Model file for the job. Use its own axes, mm. Give positions to 0.01 mm unless a question says otherwise; leave off trailing zeros. Write each loop counter-clockwise with the first axis right and the second up, starting at its lowest first coordinate (ties: lowest second). Pieces come first, ordered by that corner, then holes. Notation, with made-up numbers: (36.5, 9.25) - (81.5, 9.25) arc R21 cw to (81.5, 44.25) - close; hole circle Ø8 at (54.5, 66). An arc over 180 degrees is marked (long way). Use CSV: the item, a comma, the result in double quotes.
Solid Edge part; units mm, degrees
sketch "Sketch1" plane through (0, 0, 0) normal (0, 0, 1) x (1, 0, 0)
  line L0 (13.5, 20.7) -> (-86.5, 20.7)
  line L1 (-86.5, 20.7) -> (-86.5, -20.7)
  line L2 (-86.5, -20.7) -> (13.5, -20.7)
  line L3 (13.5, -20.7) -> (13.5, 20.7)
extrude "Protrusion1" add sketch "Sketch1" along normal blind 4
hole "Hole_1" at (-10, 10, 4) direction (0, 0, -1) diameter 3.4 end up to next
pattern_linear "Pattern1" count 2 spacing 20 along (1, 0, 0) count 2 spacing 20 along (0, -1, 0) of "Hole_1"
fillet "Round_1" radius 1.5 4 edges at (13.5, 20.7, 2) (13.5, -20.7, 2) (-86.5, -20.7, 2) (-86.5, 20.7, 2)
hole "Hole_2" at (-44.15, 10, 4) direction (0, 0, -1) diameter 3.4 end up to next
pattern_linear "Pattern3" count 2 spacing 20 along (0, -1, 0) count 2 spacing 26 along (1, 0, 0) of "Hole_2"
properties material "Aluminum, 6061-T6"
(1) Saw through at A-A, the plane y = 10. List the corners of the cut face in (x, z).
Checked values:
outline,"(-86.5, 0) - (-45.85, 0) - (-45.85, 4) - (-86.5, 4) - close; (-42.45, 0) - (-19.85, 0) - (-19.85, 4) - (-42.45, 4) - close; (-16.45, 0) - (-11.7, 0) - (-11.7, 4) - (-16.45, 4) - close; (-8.3, 0) - (8.3, 0) - (8.3, 4) - (-8.3, 4) - close; (11.7, 0) - (13.5, 0) - (13.5, 4) - (11.7, 4) - close"
(2) Saw through at C-C, the plane z = 2.8. Count the separate pieces of the cut face and the enclosed holes in it, then the cut area to 3 significant figures.
Checked values:
separate pieces,"1"
enclosed holes,"8"
area,"4,070 mm^2"
(3) Wall check: probe 1 along Y at (x, z) = (-10, 1.4); probe 2 along X at (y, z) = (10, 1.9); probe 3 along X at (y, z) = (-11.5, 3.8). Give the ranges that are in metal, low to high. Write a range as [from, to].
Checked values:
probe 1,"y = [-20.7, -11.7], [-8.3, 8.3], [11.7, 20.7]"
probe 2,"x = [-86.5, -45.85], [-42.45, -19.85], [-16.45, -11.7], [-8.3, 8.3], [11.7, 13.5]"
probe 3,"x = [-86.5, -44.95], [-43.35, -18.95], [-17.35, -10.8], [-9.2, 9.2], [10.8, 13.5]"
(4) Pull direction X, two halves, no side cores. Call faces 1 (the face through (-11.5, 9.2, 2)), 2 (the face through (-37, 0, 0)), 3 (the face through (13.5, 0, 2)): released by +X, released by -X, zero draft, split by the parting line, or undercut.
Checked values:
face 1,"undercut"
face 2,"zero draft"
face 3,"released by +X"
(5) Flat gauge pin, fed straight in: P1, Ø2, axis at x = -18.15, y = -10, coming from the -Z side. Where does the tip first touch, or does it go through?
Checked values:
P1,"passes through"
(6) Saw through at B-B, the plane x = -10. List the corners of the cut face in (y, z), then the cut area to 3 significant figures.
Checked values:
outline,"(-20.7, 0) - (-11.7, 0) - (-11.7, 4) - (-20.7, 4) - close; (-8.3, 0) - (8.3, 0) - (8.3, 4) - (-8.3, 4) - close; (11.7, 0) - (20.7, 0) - (20.7, 4) - (11.7, 4) - close"
area,"138 mm^2"
